Could you check a few things on this model? Use its own coordinates, in mm. A direction names the side the tool comes from. Give positions to 0.01 mm unless a question says otherwise; leave off trailing zeros. Order: outer loops, then holes, each group sorted by start corner. A loop starts at its lowest first (then second) coordinate and runs counter-clockwise, first axis right, second up. Notation, with made-up numbers: M 46,-18 L 79,-18 A18 ccw 79,-5 Z; hole C -37.75,72.25 d3. An arc over 180 degrees is marked long. Use a Markdown table: item, result. Add a question column.
Item 1: Suppose I cut it at B-B on y = -21. Write out the boundary of the cut face in (x, z), plus the area to 3 significant figures.
Item 2: Suppose I cut it at A-A on x = 6.5. Write out the boundary of the cut face in (y, z), plus the area to 3 significant figures.
Item 3: I'm going to push flat-ended pins straight in: pin 1 Ø1.5 at (x, z) = (-1.5, 2) entering from -Y; pin 2 Ø1.5 at (y, z) = (-145.5, 1.5) entering from -X; pin 3 Ø1.5 at (y, z) = (-100.5, 1.5) entering from +X; pin 4 Ø1.5 at (x, y) = (16, -131.5) entering from -Z. Where does each tip first touch, or does it pass through?
Item 4: For faces 1 (the face through (-2, -127, 1)), 2 (the face through (40, 2, 1)), 3 (the face through (111, -67, 1)), which set-ups out of +Z, -Z, +X, -X, +Y, -Y let a thin tool reach every point of the face, with its end or its side?
Item 5: If I drill on L1, parallel to X at y = -23.5, z = 0.7; L2, parallel to Y at x = 107, z = 1.15, over which ranges is the centre line in solid material (lowest first)? Write a range as from..to.
Autodesk Inventor part; units mm, degrees
ref_plane "YZ Plane" through (0, 0, 0) normal (1, 0, 0) x (0, 1, 0)
ref_plane "XZ Plane" through (0, 0, 0) normal (0, 1, 0) x (-1, 0, 0)
ref_plane "XY Plane" through (0, 0, 0) normal (0, 0, 1) x (1, 0, 0)
sketch "Sketch1" plane through (0, 0, 0) normal (0, 0, 1) x (1, 0, 0)
  line L0 (311.0517, -16.9965) -> (311.0486, -14.2996) construction
  line L1 (311.0486, -14.2996) -> (302.0591, -14.3097) construction
  line L2 (302.0591, -14.3097) -> (302.0622, -17.0066) construction
  line L3 (302.0622, -17.0066) -> (293.0727, -17.0167) construction
  line L4 (293.0727, -17.0167) -> (293.0696, -14.3199) construction
  line L5 (293.0696, -14.3199) -> (284.0801, -14.33) construction
  line L6 (284.0801, -14.33) -> (284.0832, -17.0268) construction
  line L7 (284.0832, -17.0268) -> (275.0937, -17.0369) construction
  line L8 (275.0937, -17.0369) -> (275.0906, -14.3401) construction
  line L9 (275.0906, -14.3401) -> (266.1012, -14.3502) construction
  line L10 (266.1012, -14.3502) -> (266.1042, -17.047) construction
  line L11 (266.1042, -17.047) -> (257.1147, -17.0571) construction
  line L12 (257.1147, -17.0571) -> (257.1117, -14.3603) construction
  line L13 (257.1117, -14.3603) -> (248.1222, -14.3704) construction
  line L14 (248.1222, -14.3704) -> (248.1252, -17.0672) construction
  line L15 (248.1252, -17.0672) -> (239.1357, -17.0773) construction
  line L16 (239.1357, -17.0773) -> (239.1327, -14.3805) construction
  line L17 (239.1327, -14.3805) -> (230.1432, -14.3906) construction
  line L18 (230.1432, -14.3906) -> (230.1462, -17.0874) construction
  line L19 (320.0411, -23.2891) -> (322.738, -23.2891) construction
  line L20 (322.738, -23.2891) -> (322.738, -32.986) construction
  line L21 (322.738, -32.986) -> (320.0411, -32.986) construction
  line L22 (320.0411, -32.986) -> (320.0411, -41.9755) construction
  line L23 (320.0411, -41.9755) -> (322.738, -41.9755) construction
  line L24 (322.738, -41.9755) -> (322.738, -50.965) construction
  line L25 (322.738, -50.965) -> (320.0411, -50.965) construction
  line L26 (320.0411, -50.965) -> (320.0411, -59.9545) construction
  line L27 (320.0411, -59.9545) -> (322.738, -59.9545) construction
  line L28 (322.738, -59.9545) -> (322.738, -68.944) construction
  line L29 (322.738, -68.944) -> (320.0411, -68.944) construction
  line L30 (320.0411, -68.944) -> (320.0411, -77.9335) construction
  line L31 (320.0411, -77.9335) -> (322.738, -77.9335) construction
  line L32 (322.738, -77.9335) -> (322.738, -86.9229) construction
  line L33 (322.738, -86.9229) -> (320.0411, -86.9229) construction
  line L34 (320.0411, -86.9229) -> (320.0411, -95.9124) construction
  line L35 (320.0411, -95.9124) -> (322.738, -95.9124) construction
  line L36 (322.738, -95.9124) -> (322.738, -104.9019) construction
  line L37 (322.738, -104.9019) -> (320.0411, -104.9019) construction
  line L38 (322.738, -113.8914) -> (323.0503, -123.1532) construction
  line L39 (323.0503, -123.1532) -> (328.4284, -122.9718) construction
  line L40 (328.4284, -122.9718) -> (328.4284, -131.9613) construction
  line L41 (328.4284, -131.9613) -> (331.1252, -131.9613) construction
  line L42 (331.1252, -131.9613) -> (331.1252, -140.9508) construction
  line L43 (331.1252, -140.9508) -> (328.4284, -140.9508) construction
  line L44 (328.4284, -140.9508) -> (328.4284, -147.2435) construction
  line L45 (318.4284, -147.2435) -> (318.4284, -149.9403) construction
  line L46 (318.4284, -149.9403) -> (308.4284, -149.9403) construction
  line L47 (308.4284, -149.9403) -> (308.4284, -147.2435) construction
  line L48 (308.4284, -147.2435) -> (298.4284, -147.2435) construction
  line L49 (298.4284, -147.2435) -> (298.4284, -149.9403) construction
  line L50 (298.4284, -149.9403) -> (288.4284, -149.9403) construction
  line L51 (288.4284, -149.9403) -> (288.4284, -147.2435) construction
  line L52 (288.4284, -147.2435) -> (278.4284, -147.2435) construction
  line L53 (278.4284, -147.2435) -> (278.4284, -149.9403) construction
  line L54 (278.4284, -149.9403) -> (268.4284, -149.9403) construction
  line L55 (268.4284, -149.9403) -> (268.4284, -147.2435) construction
  line L56 (268.4284, -147.2435) -> (258.4284, -147.2435) construction
  line L57 (258.4284, -147.2435) -> (258.4284, -149.9403) construction
  line L58 (258.4284, -149.9403) -> (248.4284, -149.9403) construction
  line L59 (248.4284, -149.9403) -> (248.4284, -147.2435) construction
  line L60 (248.4284, -147.2435) -> (239.4389, -147.2435) construction
  line L61 (239.4389, -147.2435) -> (239.4389, -149.9403) construction
  line L62 (239.4389, -149.9403) -> (230.4494, -149.9403) construction
  line L63 (230.4494, -149.9403) -> (230.4494, -147.2435) construction
  line L64 (218.4599, -140.9508) -> (218.4599, -131.9613) construction
  line L65 (218.4599, -131.9613) -> (221.1567, -131.9613) construction
  line L66 (221.1567, -131.9613) -> (221.1567, -122.9718) construction
  line L67 (221.1567, -122.9718) -> (218.4599, -122.9718) construction
  line L68 (218.4599, -122.9718) -> (218.4599, -113.9823) construction
  line L69 (218.4599, -113.9823) -> (221.1567, -113.9823) construction
  line L70 (221.1567, -113.9823) -> (221.1567, -104.9929) construction
  line L71 (221.1567, -104.9929) -> (218.4599, -104.9929) construction
  line L72 (218.4599, -104.9929) -> (218.4599, -96.0034) construction
  line L73 (218.4599, -96.0034) -> (221.1567, -96.0034) construction
  line L74 (221.1567, -96.0034) -> (221.1567, -87.0139) construction
  line L75 (221.1567, -87.0139) -> (218.4599, -87.0139) construction
  line L76 (218.4599, -87.0139) -> (218.4599, -78.0244) construction
  line L77 (218.4599, -78.0244) -> (221.1567, -78.0244) construction
  line L78 (221.1567, -78.0244) -> (221.1567, -69.0349) construction
  line L79 (221.1567, -69.0349) -> (218.4599, -69.0349) construction
  line L80 (218.4599, -69.0349) -> (218.4599, -60.0454) construction
  line L81 (218.4599, -60.0454) -> (221.1567, -60.0454) construction
  line L82 (221.1567, -60.0454) -> (221.1567, -51.0559) construction
  line L83 (221.1567, -51.0559) -> (218.4599, -51.0559) construction
  line L84 (218.4599, -51.0559) -> (218.4599, -42.0664) construction
  line L85 (218.4599, -42.0664) -> (221.1567, -42.0664) construction
  line L86 (221.1567, -42.0664) -> (221.1567, -33.0769) construction
  line L87 (221.1567, -33.0769) -> (218.4599, -33.0769) construction
  line L88 (218.4599, -33.0769) -> (218.4599, -24.0874) construction
  line L89 (218.4599, -24.0874) -> (221.1567, -24.0874) construction
  line L90 (221.1567, -24.0874) -> (221.1567, -17.0874) construction
  line L91 (320.0411, -104.9019) -> (320.0411, -113.8914) construction
  line L92 (320.0411, -113.8914) -> (322.738, -113.8914) construction
  line L93 (318.4284, -147.2435) -> (328.4284, -147.2435) construction
  line L94 (221.1567, -17.0874) -> (230.1462, -17.0874) construction
  line L95 (221.4599, -147.2435) -> (230.4494, -147.2435) construction
  line L96 (311.0517, -16.9965) -> (320.0411, -16.9965) construction
  line L97 (320.0411, -16.9965) -> (320.0411, -23.2891) construction
  line L98 (221.4599, -147.2435) -> (221.4599, -140.9508) construction
  line L99 (218.4599, -140.9508) -> (221.4599, -140.9508) construction
  line L100 (0, 0) -> (10, 0)
  line L101 (10, 0) -> (10, 3)
  line L102 (10, 3) -> (20, 3)
  line L103 (20, 3) -> (20, 0)
  line L104 (20, 0) -> (30, 0)
  line L105 (30, 0) -> (30, 3)
  line L106 (30, 3) -> (40, 3)
  line L107 (40, 3) -> (40, 0)
  line L108 (40, 0) -> (50, 0)
  line L109 (50, 0) -> (50, 3)
  line L110 (50, 3) -> (60, 3)
  line L111 (60, 3) -> (60, 0)
  line L112 (60, 0) -> (70, 0)
  line L113 (70, 0) -> (70, 3)
  line L114 (70, 3) -> (80, 3)
  line L115 (80, 3) -> (80, 0)
  line L116 (80, 0) -> (90, 0)
  line L117 (90, 0) -> (90, 3)
  line L118 (90, 3) -> (100, 3)
  line L119 (100, 3) -> (100, 0)
  line L120 (100, 0) -> (110, 0)
  line L121 (110, 0) -> (110, -7)
  line L122 (110, -7) -> (113, -7)
  line L123 (113, -7) -> (113, -17)
  line L124 (113, -17) -> (110, -17)
  line L125 (110, -17) -> (110, -27)
  line L126 (110, -27) -> (113, -27)
  line L127 (113, -27) -> (113, -37)
  line L128 (113, -37) -> (110, -37)
  line L129 (110, -37) -> (110, -47)
  line L130 (110, -47) -> (113, -47)
  line L131 (113, -47) -> (113, -57)
  line L132 (113, -57) -> (110, -57)
  line L133 (110, -57) -> (110, -67)
  line L134 (110, -67) -> (113, -67)
  line L135 (113, -67) -> (113, -77)
  line L136 (113, -77) -> (110, -77)
  line L137 (110, -77) -> (110, -87)
  line L138 (110, -87) -> (113, -87)
  line L139 (113, -87) -> (113, -97)
  line L140 (113, -97) -> (110, -97)
  line L141 (110, -97) -> (110, -107)
  line L142 (110, -107) -> (113, -107)
  line L143 (113, -107) -> (113, -117)
  line L144 (113, -117) -> (110, -117)
  line L145 (110, -117) -> (110, -127)
  line L146 (110, -127) -> (113, -127)
  line L147 (113, -127) -> (113, -137)
  line L148 (113, -137) -> (110, -137)
  line L149 (110, -137) -> (110, -144)
  line L150 (110, -144) -> (100, -144)
  line L151 (100, -144) -> (100, -147)
  line L152 (100, -147) -> (90, -147)
  line L153 (90, -147) -> (90, -144)
  line L154 (90, -144) -> (80, -144)
  line L155 (80, -144) -> (80, -147)
  line L156 (80, -147) -> (70, -147)
  line L157 (70, -147) -> (70, -144)
  line L158 (70, -144) -> (60, -144)
  line L159 (60, -144) -> (60, -147)
  line L160 (60, -147) -> (50, -147)
  line L161 (50, -147) -> (50, -144)
  line L162 (50, -144) -> (40, -144)
  line L163 (40, -144) -> (40, -147)
  line L164 (40, -147) -> (30, -147)
  line L165 (30, -147) -> (30, -144)
  line L166 (30, -144) -> (20, -144)
  line L167 (20, -144) -> (20, -147)
  line L168 (20, -147) -> (10, -147)
  line L169 (10, -147) -> (10, -144)
  line L170 (10, -144) -> (0, -144)
  line L171 (0, -144) -> (0, -137)
  line L172 (0, -137) -> (-3, -137)
  line L173 (-3, -137) -> (-3, -127)
  line L174 (-3, -127) -> (0, -127)
  line L175 (0, -127) -> (0, -117)
  line L176 (0, -117) -> (-3, -117)
  line L177 (-3, -117) -> (-3, -107)
  line L178 (-3, -107) -> (0, -107)
  line L179 (0, -107) -> (0, -97)
  line L180 (0, -97) -> (-3, -97)
  line L181 (-3, -97) -> (-3, -87)
  line L182 (-3, -87) -> (0, -87)
  line L183 (0, -87) -> (0, -77)
  line L184 (0, -77) -> (-3, -77)
  line L185 (-3, -77) -> (-3, -67)
  line L186 (-3, -67) -> (0, -67)
  line L187 (0, -67) -> (0, -57)
  line L188 (0, -57) -> (-3, -57)
  line L189 (-3, -57) -> (-3, -47)
  line L190 (-3, -47) -> (0, -47)
  line L191 (0, -47) -> (0, -37)
  line L192 (0, -37) -> (-3, -37)
  line L193 (-3, -37) -> (-3, -27)
  line L194 (-3, -27) -> (0, -27)
  line L195 (0, -27) -> (0, -17)
  line L196 (0, -17) -> (-3, -17)
  line L197 (-3, -17) -> (-3, -7)
  line L198 (-3, -7) -> (0, -7)
  line L199 (0, -7) -> (0, 0)
  dimension "d263" = 8.9895
  dimension "d264" = 7
  dimension "d265" = 10
  dimension "d266" = 3
  dimension "d267" = 10
  dimension "d268" = 10
  dimension "d269" = 10
  dimension "d270" = 10
  dimension "d271" = 10
  dimension "d272" = 10
  dimension "d273" = 10
  dimension "d274" = 10
  dimension "d275" = 10
  dimension "d276" = 10
  dimension "d277" = 7
  dimension "d278" = 3
  dimension "d279" = 10
  dimension "d280" = 10
  dimension "d281" = 10
  dimension "d282" = 10
  dimension "d283" = 10
  dimension "d284" = 10
  dimension "d285" = 10
  dimension "d286" = 10
  dimension "d287" = 10
  dimension "d288" = 10
  dimension "d289" = 10
  dimension "d290" = 10
  dimension "d291" = 10
  dimension "d292" = 7
  dimension "d293" = 3
  dimension "d294" = 3
  dimension "d295" = 110
  dimension "d296" = 144
  dimension "d297" = 3
  dimension "d298" = 3
  dimension "d299" = 3
  dimension "d300" = 3
  dimension "d301" = 3
extrude "Extrusion1" add sketch "Sketch1" along normal blind 3
properties part number "cara_posterior"
Findings below:
| question | item | result |
|---|---|---|
| 1 | outline | M 0,0 L 110,0 L 110,3 L 0,3 Z |
| 1 | area | 330 mm^2 |
| 2 | outline | M -144,0 L 0,0 L 0,3 L -144,3 Z |
| 2 | area | 432 mm^2 |
| 3 | pin 1 | stops at y = -137 |
| 3 | pin 2 | stops at x = 10 |
| 3 | pin 3 | stops at x = 110 |
| 3 | pin 4 | stops at z = 0 |
| 4 | face 1 | +Z, -Z, -X |
| 4 | face 2 | +Z, -Z, +Y |
| 4 | face 3 | +Z, -Z, +X |
| 5 | L1 | x = 0..110 |
| 5 | L2 | y = -144..0 |
